Here's how the part is built. I have some questions about the finished solid (model axes, mm). Coordinates: 2 decimals unless noted, no trailing zeros. Write each loop counter-clockwise with the first axis right and the second up, starting at its lowest first coordinate (ties: lowest second). Pieces come first, ordered by that corner, then holes.
Autodesk Inventor part; units mm, degrees
ref_plane "Work Plane1" through (3.81, 0, 0) normal (1, 0, 0) x (0, 1, 0)
sketch "Sketch2" plane through (3.81, 0, 0) normal (1, 0, 0) x (0, 1, 0)
  line L0 (-38.5826, 0) -> (38.5826, 0)
  line L1 (0, 38.5826) -> (0, -38.5826)
  point P0 (0, 0)
  point P1 (0, 27.559)
  point P2 (0, -27.559)
  dimension "d6" = 55.118
  dimension "d7" = 27.559
sketch "Sketch1" plane through (0, 0, 0) normal (0, 0, 1) x (1, 0, 0)
  circle A0 centre (0, 0) radius 2.3749
  dimension "d0" = 4.7498
extrude "Extrusion1" add sketch "Sketch1" along normal mid plane 60.198
chamfer "Chamfer1" distance 0.254 angle 45 2 edges at (-2.3749, 0, 30.099) (-2.3749, 0, -30.099)
hole "Hole1" at (3.81, 0, 27.559) at (3.81, 0, -27.559) direction (-1, 0, 0) diameter 1.5748 end through all
properties part number "J005527" material "ALUMINUM, 6061-T651"
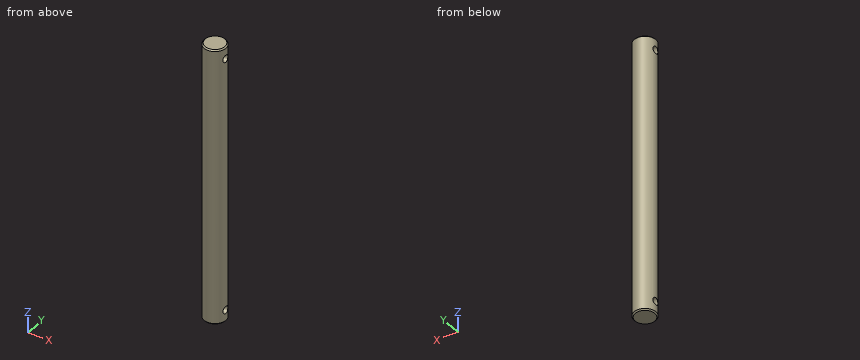
1) Imagine slicing it at B-B on z = -8.5. Please give me the cut outline in (x, y), then the cut area to 3 significant figures.
Values follow:
outline: circle Ø4.75 at (0, 0)
area: 17.7 mm2
2) Will this pin go through, and if not, where does the flat tip stop? pin 1 (0.9 mm diameter, centred on y = 0, z = 27.559, fed in from +X).
Values follow:
pin 1: passes through
3) Imagine slicing it at C-C on x = -0.6. Count the separate pieces of the cut face and the enclosed holes in it, then the cut area to 3 significant figures.
Values follow:
separate pieces: 1
enclosed holes: 2
area: 273 mm2
4) I need wall thicknesses on probe 1 along Z at (x, y) = (-1.35, 0); probe 2 along Z at (x, y) = (-0.3, -0.4); probe 3 along Y at (x, z) = (-0.1, 25). Which ranges of each line are inside material? Lowest first, please.
Values follow:
probe 1: z = -30.1 to -28.35, -26.77 to 26.77, 28.35 to 30.1
probe 2: z = -30.1 to -28.24, -26.88 to 26.88, 28.24 to 30.1
probe 3: y = -2.37 to 2.37
5) Imagine slicing it at A-A on y = 0. Please give me the cut outline in (x, z) (3 decimals).
Values follow:
outline: (-2.375, -29.845) - (-2.121, -30.099) - (2.121, -30.099) - (2.375, -29.845) - (2.375, -28.346) - (-2.375, -28.346) - close; (-2.375, -26.772) - (2.375, -26.772) - (2.375, 26.772) - (-2.375, 26.772) - close; (-2.375, 28.346) - (2.375, 28.346) - (2.375, 29.845) - (2.121, 30.099) - (-2.121, 30.099) - (-2.375, 29.845) - close
